The listing builds one solid part. Answer for the finished solid, in the listing's coordinates (mm). Face numbers are marked on the shaded views. A direction names the side the tool comes from. Coordinates: 2 decimals unless noted, no trailing zeros. Loops run counter-clockwise (first coordinate to the right, second up) from the corner with the lowest first, then second, coordinate; pieces in that order, holes last. Notation, with made-up numbers: (11, 13.5) -> (35, 13.5) arc R10 ccw to (35, 31.5) -> close; hole circle Ø2 at (23, 9). An arc over 180 degrees is marked (long way). Answer in a Markdown table with one row per item.
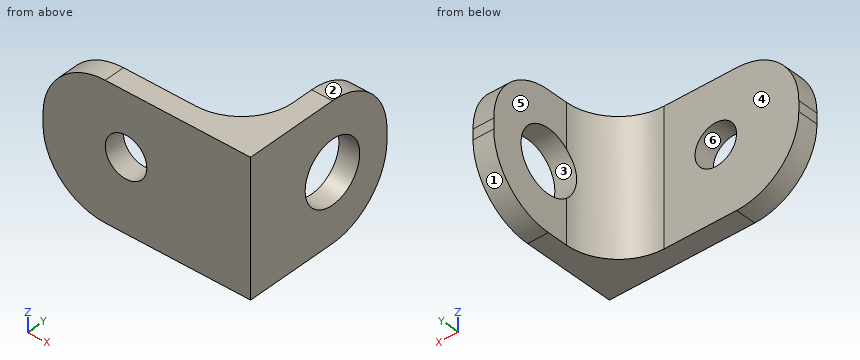
Autodesk Inventor part; units mm, degrees
ref_plane "YZ Plane" through (0, 0, 0) normal (1, 0, 0) x (0, 1, 0)
ref_plane "XZ Plane" through (0, 0, 0) normal (0, 1, 0) x (-1, 0, 0)
ref_plane "XY Plane" through (0, 0, 0) normal (0, 0, 1) x (1, 0, 0)
sketch "Sketch1" plane through (0, 0, 0) normal (0, 0, 1) x (1, 0, 0)
  line L0 (0, 0) -> (-20, 0)
  line L1 (-20, 0) -> (-20, 2)
  line L2 (-20, 2) -> (0, 2)
  line L3 (0, 2) -> (0, 0)
  line L4 (0, 0) -> (-2, 0)
  line L5 (-2, 0) -> (-2, 15)
  line L6 (-2, 15) -> (0, 15)
  line L7 (0, 15) -> (0, 0)
  point P0 (-2, 2)
  dimension "d0" = 20
  dimension "d1" = 2
  dimension "d2" = 2
  dimension "d3" = 15
extrude "Extrusion1" add sketch "Sketch1" along normal blind 13
fillet "Fillet1" radius 5 1 edges at (-2, 2, 6.5)
fillet "Fillet2" radius 6 4 edges at (-1, 15, 13) (-1, 15, 0) (-20, 1, 13) (-20, 1, 0)
sketch "Sketch2" plane through (0, 0, 13) normal (1, 0, 0) x (0, 0, -1)
  line L0 (13, 0) -> (0, 0)
  line L1 (6.5, 0) -> (6.5, 9)
  circle A0 centre (6.5, 9) radius 3
  dimension "d8" = 9
  dimension "d9" = 6
extrude "Extrusion2" cut sketch "Sketch2" against normal blind 13
sketch "Sketch3" plane through (0, 0, 0) normal (0, -1, 0) x (1, 0, 0)
  line L0 (0, 7) -> (-2, 7)
  line L1 (0, 7) -> (-12, 7)
  circle A0 centre (-12, 7) radius 2
  point P0 (0, 0)
  dimension "d12" = 12
  dimension "d13" = 4
extrude "Extrusion3" cut sketch "Sketch3" against normal blind 13
properties part number "prependicular"
Item 1: A cutting plane is placed at B-B, the plane y = 8. Determine the outline of the cut face in (x, z).
Findings below:
| item | result |
|---|---|
| outline | (-2, 0) -> (0, 0) -> (0, 3.67) -> (-2, 3.67) -> close; (-2, 9.33) -> (0, 9.33) -> (0, 13) -> (-2, 13) -> close |
Item 2: Flat-ended cylindrical pins translate along their axes: pin 1 Ø1.5 at (y, z) = (6, 9.5) entering from -X; pin 2 Ø4 at (y, z) = (10, 4) entering from -X; pin 3 Ø6.5 at (x, z) = (-16.5, 7.5) entering from +Y. Find the tip coordinate at first contact, or state that the pin passes through.
Findings below:
| item | result |
|---|---|
| pin 1 | stops at x = -2.32 |
| pin 2 | stops at x = -2 |
| pin 3 | stops at y = 2 |
Item 3: Determine the mould class of the marked faces 1, 2, 3 and 4 for opening direction Z: +Z half, -Z half, draft (parallel to the pull), parting line (faces both ways), or undercut.
Findings below:
| item | result |
|---|---|
| face 1 | -Z half |
| face 2 | +Z half |
| face 3 | undercut |
| face 4 | draft |
Item 4: Find the intervals of material crossed by probe 1 along Z at (x, y) = (-0.8, 9); probe 2 along Z at (x, y) = (-12, 1.45); probe 3 along Y at (x, z) = (-13, 2), in increasing order.
Findings below:
| item | result |
|---|---|
| probe 1 | z = 0 to 3.5, 9.5 to 13 |
| probe 2 | z = 0 to 5, 9 to 13 |
| probe 3 | y = 0 to 2 |
Item 5: A cutting plane is placed at C-C, the plane z = 6.5. Determine the outline of the cut face in (x, y), plus the area to 3 significant figures.
Findings below:
| item | result |
|---|---|
| outline | (-20, 0) -> (-13.94, 0) -> (-13.94, 2) -> (-20, 2) -> close; (-10.06, 0) -> (0, 0) -> (0, 6) -> (-2.1, 6) arc R5 cw to (-7, 2) -> (-10.06, 2) -> close; (-2, 12) -> (0, 12) -> (0, 15) -> (-2, 15) -> close |
| area | 51.6 mm2 |
Item 6: A cutting plane is placed at A-A, the plane x = -12. Determine the outline of the cut face in (y, z).
Findings below:
| item | result |
|---|---|
| outline | (0, 0) -> (2, 0) -> (2, 5) -> (0, 5) -> close; (0, 9) -> (2, 9) -> (2, 13) -> (0, 13) -> close |
Item 7: A tool of negligible diameter and unlimited length cuts with its end or side. For the marked faces 5 and 6, from which of +Z, -Z, +X, -X, +Y, -Y can it reach the whole face along a straight path? Write none if from no direction.
Findings below:
| item | result |
|---|---|
| face 5 | +Z, -Z, -X, +Y |
| face 6 | +Y, -Y |
Item 8: A cutting plane is placed at D-D, the plane z = 4.5. Determine the outline of the cut face in (x, y).
Findings below:
| item | result |
|---|---|
| outline | (-19.81, 0) -> (0, 0) -> (0, 6.76) -> (-2.01, 6.76) arc R5 cw to (-7, 2) -> (-19.81, 2) -> close; (-2, 11.24) -> (0, 11.24) -> (0, 14.81) -> (-2, 14.81) -> close |
